For this review, take the finished solid that the model builds, in its own axes (mm). Give positions to 0.01 mm unless a question says otherwise; leave off trailing zeros. Write each loop counter-clockwise with the first axis right and the second up, starting at its lowest first coordinate (ties: lowest second). Pieces come first, ordered by that corner, then holes. Notation, with made-up numbers: (-6, -31) -> (43, -31) arc R24 cw to (43, 4) -> close; hole circle Ø5 at (1, -15). An arc over 180 degrees is marked (long way). Return JSON: item names as keys, results as strings.
from build123d import *

# Parameters (mm, degrees)
F0_R     = 2.5
F1_DEPTH = 2
F2_SIZE  = 4


with BuildPart() as f1:
    # F0 (on Front) → F1 (new body)
    with BuildSketch(Plane.XZ):
        Polygon((-110, 38), (-110, 0), (0, 0), (0, 38), (-26, 38), (-26, 80), (-84, 80), (-84, 38), align=None)
        with Locations((-101, 9)):
            Circle(F0_R, mode=Mode.SUBTRACT)
        with Locations((-101, 29)):
            Circle(F0_R, mode=Mode.SUBTRACT)
        with Locations((-9, 9)):
            Circle(F0_R, mode=Mode.SUBTRACT)
        with Locations((-9, 29)):
            Circle(F0_R, mode=Mode.SUBTRACT)
        with Locations((-75, 71)):
            Circle(F0_R, mode=Mode.SUBTRACT)
        with Locations((-55, 71)):
            Circle(F0_R, mode=Mode.SUBTRACT)
        with Locations((-35, 71)):
            Circle(F0_R, mode=Mode.SUBTRACT)
    extrude(amount=F1_DEPTH)

    # F2
    f2_edges = [f1.edges().sort_by_distance(p)[0] for p in [
        (-26, -1, 80),
        (-84, -1, 80),
        (0, -1, 38),
        (-110, -1, 38),
        (0, -1, 0),
        (-110, -1, 0),
    ]]
    chamfer(f2_edges, length=F2_SIZE)


solid = f1.part
1. Add section D-D, the plane z = 60. State the section outline as (x, y) points.
Results found:
{"outline": "(-84, -2) -> (-26, -2) -> (-26, 0) -> (-84, 0) -> close"}
2. For pin 1 (0.6 mm diameter, centred on x = -12.5, y = -1.5, fed in from +Z); pin 2 (1 mm diameter, centred on y = -0.5, z = 54.5, fed in from +X); pin 3 (4 mm diameter, centred on x = -101, z = 9, fed in from -Y); pin 4 (0.6 mm diameter, centred on y = -1, z = 51, fed in from -X), all flat-tipped, find the tip position at first contact; note any pin that passes through.
Results found:
{"pin 1": "stops at z = 38", "pin 2": "stops at x = -26", "pin 3": "passes through", "pin 4": "stops at x = -84"}
3. Add section A-A, the plane x = -101. State the section outline as (y, z) points.
Results found:
{"outline": "(-2, 0) -> (0, 0) -> (0, 6.5) -> (-2, 6.5) -> close; (-2, 11.5) -> (0, 11.5) -> (0, 26.5) -> (-2, 26.5) -> close; (-2, 31.5) -> (0, 31.5) -> (0, 38) -> (-2, 38) -> close"}
4. To check wall thickness, follow probe 1 along Z at (x, y) = (-101, -1); probe 2 along Z at (x, y) = (-10, -1.8); probe 3 along X at (y, z) = (-0.2, 70.5). State the ranges of each line that lie inside material, in increasing order.
Results found:
{"probe 1": "z = 0 to 6.5, 11.5 to 26.5, 31.5 to 38", "probe 2": "z = 0 to 6.71, 11.29 to 26.71, 31.29 to 38", "probe 3": "x = -84 to -77.45, -72.55 to -57.45, -52.55 to -37.45, -32.55 to -26"}
5. Add section B-B, the plane y = -1. State the section outline as (x, z) points, plus the area to 3 significant figures.
Results found:
{"outline": "(-110, 4) -> (-106, 0) -> (-4, 0) -> (0, 4) -> (0, 34) -> (-4, 38) -> (-26, 38) -> (-26, 76) -> (-30, 80) -> (-80, 80) -> (-84, 76) -> (-84, 38) -> (-106, 38) -> (-110, 34) -> close; hole circle Ø5 at (-101, 9); hole circle Ø5 at (-101, 29); hole circle Ø5 at (-75, 71); hole circle Ø5 at (-55, 71); hole circle Ø5 at (-35, 71); hole circle Ø5 at (-9, 9); hole circle Ø5 at (-9, 29)", "area": "6,430 mm²"}
6. The part is to be moulded in two halves that separate along X. For faces 1 (the flat face through (-2, -1, 36)), 2 (the cylindrical face through (-99.85, -0.99, 6.78)), 3 (the flat face through (-56, -2, 32)), say which applies: +X half, -X half, draft (parallel to the pull), parting line (faces both ways), or undercut.
Results found:
{"face 1": "+X half", "face 2": "undercut", "face 3": "draft"}
7. Add section C-C, the plane x = -75. State the section outline as (y, z) points, plus the area to 3 significant figures.
Results found:
{"outline": "(-2, 0) -> (0, 0) -> (0, 68.5) -> (-2, 68.5) -> close; (-2, 73.5) -> (0, 73.5) -> (0, 80) -> (-2, 80) -> close", "area": "150 mm²"}
